Model file for the job. Use its own axes, mm. A direction names the side the tool comes from. Round coordinates to 2 decimals unless told otherwise and drop trailing zeros. Loops run counter-clockwise (first coordinate to the right, second up) from the corner with the lowest first, then second, coordinate; pieces in that order, holes last. Notation, with made-up numbers: (70, -38) -> (121, -38) arc R29 ccw to (121, -1) -> close; hole circle Ø2 at (17, 58.25). An arc over 180 degrees is marked (long way). Use a Markdown table: item, result. Add a question column.
```python
from build123d import *

# Parameters (mm, degrees)
SKETCH_1_R      = 1.5
EXTRUDE_1_DEPTH = 2.5
SKETCH_2_R      = 5
EXTRUDE_2_DEPTH = 5
SKETCH_3_W      = 5
SKETCH_3_H      = 6
EXTRUDE_3_DEPTH = 30


with BuildPart() as part:
    # 草图1 → 凸台-拉伸1 (new body)
    with BuildSketch(Plane(origin=(0, 0, 0), x_dir=(0, 0, -1), z_dir=(1, 0, 0))):
        Circle(SKETCH_1_R)
    extrude(amount=EXTRUDE_1_DEPTH)

    # 草图2 → 凸台-拉伸2 (add)
    with BuildSketch(Plane(origin=(2.5, 0, 0), x_dir=(0, 0, -1), z_dir=(1, 0, 0))):
        Circle(SKETCH_2_R)
    extrude(amount=EXTRUDE_2_DEPTH)

    # 草图3 → 凸台-拉伸3 (add)
    with BuildSketch(Plane(origin=(0, 0, 0), x_dir=(1, 0, 0), z_dir=(0, 1, 0))):
        with Locations((5, 0)):
            Rectangle(SKETCH_3_W, SKETCH_3_H)
    extrude(amount=-EXTRUDE_3_DEPTH)


solid = part.part
```
1) Pin check, flat tips, straight feed: pin 1 Ø2.5 at (x, y) = (6, -20) entering from -Z; pin 2 Ø4 at (x, y) = (4.5, -14) entering from +Z; pin 3 Ø4 at (x, z) = (1.5, -2.5) entering from +Y. Stop position of each tip, or through.
2) Cut at B-B on z = 0. Write the cut outline in (x, y).
3) Wall check: probe 1 along X at (y, z) = (-3, -1.5); probe 2 along Z at (x, y) = (3, 4). Give the ranges that are in metal, low to high. Write a range as from..to.
4) Tool access for faces 1 (the face through (5, -17, 3)), 2 (the face through (5, -17, -3)), 3 (the face through (1.23, 0.07, 1.5)): list every direction of +Z, -Z, +X, -X, +Y, -Y with a clear straight run to the whole face (end or side of a thin tool).
5) Cut at A-A on y = 0. Write the cut outline in (x, z).
6) Cut at D-D on y = -26.5. Write the cut outline in (x, z), and give its area (3 significant figures).
7) Cut at C-C on x = 3.5. Write the cut outline in (y, z), and give its area (3 significant figures).
Established:
| question | item | result |
|---|---|---|
| 1 | pin 1 | stops at z = -3 |
| 1 | pin 2 | stops at z = 3 |
| 1 | pin 3 | stops at y = 4.94 |
| 2 | outline | (0, -1.5) -> (2.5, -1.5) -> (2.5, -30) -> (7.5, -30) -> (7.5, 5) -> (2.5, 5) -> (2.5, 1.5) -> (0, 1.5) -> close |
| 3 | probe 1 | x = 2.5..7.5 |
| 3 | probe 2 | z = -3..3 |
| 4 | face 1 | +Z, +X, -X, -Y |
| 4 | face 2 | -Z, +X, -X, -Y |
| 4 | face 3 | -X |
| 5 | outline | (0, -1.5) -> (2.5, -1.5) -> (2.5, -5) -> (7.5, -5) -> (7.5, 5) -> (2.5, 5) -> (2.5, 1.5) -> (0, 1.5) -> close |
| 6 | outline | (2.5, -3) -> (7.5, -3) -> (7.5, 3) -> (2.5, 3) -> close |
| 6 | area | 30.0 mm^2 |
| 7 | outline | (-30, -3) -> (-4, -3) arc R5 ccw (long way) to (-4, 3) -> (-30, 3) -> close |
| 7 | area | 230 mm^2 |
